For this review, take the finished solid that the model builds, in its own axes (mm). A direction names the side the tool comes from. Give positions to 0.01 mm unless a question says otherwise; leave off trailing zeros. Loops run counter-clockwise (first coordinate to the right, second up) from the corner with the lowest first, then second, coordinate; pieces in that order, holes last. Notation, with made-up numbers: (35.25, -13.5) -> (54.25, -13.5) arc R14 ccw to (54.25, 12.5) -> close; hole circle Ø10 at (42.25, 53.25). An arc over 180 degrees is marked (long way). Answer as CSV lines item,"result". Start each with the question number.
Item 1: Add section B-B on y = -48.5. State the section outline as (x, z) points.
Item 2: The part is to be moulded in two halves that separate along X. For faces 1 (the face through (-9.29, -7.75, 37.81)), 2 (the face through (31.75, -1, 31)), 3 (the face through (0.444, -40.684, 14.155)), 4 (the face through (5.52, 0.07, 20.81)), say which applies: +X half, -X half, draft (parallel to the pull), parting line (faces both ways), or undercut.
Item 3: For L1, parallel to Y at x = -16.5, z = 54; L2, parallel to Y at x = -24, z = 48.5; L3, parallel to Y at x = -24, z = 37.5, list the stretches that pass through material, from the lowest coordinate up. Write a range as from..to.
Item 4: Add section A-A on x = 21.5. State the section outline as (y, z) points (3 decimals), plus the area to 3 significant figures.
Item 5: Add section C-C on z = 33. State how many separate pieces and enclosed holes the cut face has, plus the area to 3 significant figures.
Item 6: Clearance check with flat-ended pins moving along their axes: P1, Ø1.5, axis at x = -20.5, y = 43.5, coming from the +Z side; P2, Ø6, axis at x = -11.5, z = 42.5, coming from the -Y side. State where each tip first meets the part, or that it passes through.
Item 7: Machinability: for faces 5 (the face through (0.444, -60.18, 25.546)), 6 (the face through (12, 4, 63.5)), 7 (the face through (5.662, 50.867, 20.915)), which of the approach directions +Z, -Z, +X, -X, +Y, -Y give a long, thin tool a straight path to every point of the face, cutting with its end or side? Answer none if there is none.
```python
from build123d import *

# Parameters (mm, degrees)
F0_W     = 63.5
F0_H     = 139.7
F1_DEPTH = 63.5
F3_DEPTH = 139.7
F4_R     = 7.9375
F5_DEPTH = 41.275
F6_R     = 3.175
F8_DEPTH = 63.5
F9_R     = 3.175


with BuildPart() as f1:
    # F0 (on Top) → F1 (new body)
    with BuildSketch(Plane.XY):
        Rectangle(F0_W, F0_H)
    extrude(amount=F1_DEPTH)

    # F2 (on face) → F3 (cut, through all)
    with BuildSketch(Plane.XZ.offset(69.85)):
        Polygon((-31.75, 63.5), (-31.75, 44.45), (-6.35, 63.5), align=None)
    extrude(amount=-F3_DEPTH, mode=Mode.SUBTRACT)

    # F4 (on face) → F5 (cut)
    with BuildSketch(Plane(origin=(-32.766, 0, 43.688), x_dir=(0.8, 0, 0.6), z_dir=(-0.6, 0, 0.8))):
        with Locations((17.145, 50.8)):
            Circle(F4_R)
        with Locations((17.05919, 25.400145)):
            Circle(F4_R)
        with Locations((16.973379, 0.00029)):
            Circle(F4_R)
        with Locations((16.887569, -25.399565)):
            Circle(F4_R)
    extrude(amount=-F5_DEPTH, mode=Mode.SUBTRACT)

    # F6
    f6_edges = [f1.edges().sort_by_distance(p)[0] for p in [
        (-0.840945, -25.399565, 16.038041),
        (-0.772297, 0.00029, 16.089528),
        (-0.703648, 25.400145, 16.141014),
        (-0.635, 50.8, 16.1925),
    ]]
    fillet(f6_edges, radius=F6_R)

    # F7 (on face) → F8 (cut, through all)
    with BuildSketch(Plane.YZ.offset(31.75)):
        Polygon((-69.85, 63.5), (-69.85, 39.356078), (-48.414039, 8.742354), (-32.809193, 19.668985), (-63.5, 63.5), align=None)
    extrude(amount=-F8_DEPTH, mode=Mode.SUBTRACT)

    # F9
    f9_edges = [f1.edges().sort_by_distance(p)[0] for p in [
        (0, -32.809193, 19.668985),
        (0, -48.414039, 8.742354),
    ]]
    fillet(f9_edges, radius=F9_R)


solid = f1.part
```
Computed values:
1,outline,"(-31.75, 0) -> (31.75, 0) -> (31.75, 10.11) -> (-31.75, 10.11) -> close; (-31.75, 42.08) -> (31.75, 42.08) -> (31.75, 63.5) -> (-6.35, 63.5) -> (-31.75, 44.45) -> close"
2,face 1,"undercut"
2,face 2,"+X half"
2,face 3,"draft"
2,face 4,"undercut"
3,L1,"-56.85..-32.99, -17.81..-7.62, 7.62..17.76, 33.04..43.13, 58.47..69.85"
3,L2,"-53..-29.16, -21.63..-3.6, 3.6..21.97, 28.83..47.56, 54.04..69.85"
3,L3,"-69.85..-68.55, -45.29..69.85"
4,outline,"(-69.85, 0) -> (69.85, 0) -> (69.85, 63.5) -> (-63.5, 63.5) -> (-34.63, 22.27) arc R3.175 cw to (-35.41, 17.848) -> (-45.813, 10.563) arc R3.175 cw to (-50.235, 11.343) -> (-69.85, 39.356) -> close"
4,area,"7,930 mm²"
5,separate pieces,"2"
5,enclosed holes,"4"
5,area,"6,400 mm²"
6,P1,"z = 53.27"
6,P2,"y = -50.9"
7,face 5,"+X, -X"
7,face 6,"+Z, +X, -X, +Y, -Y"
7,face 7,"none"
